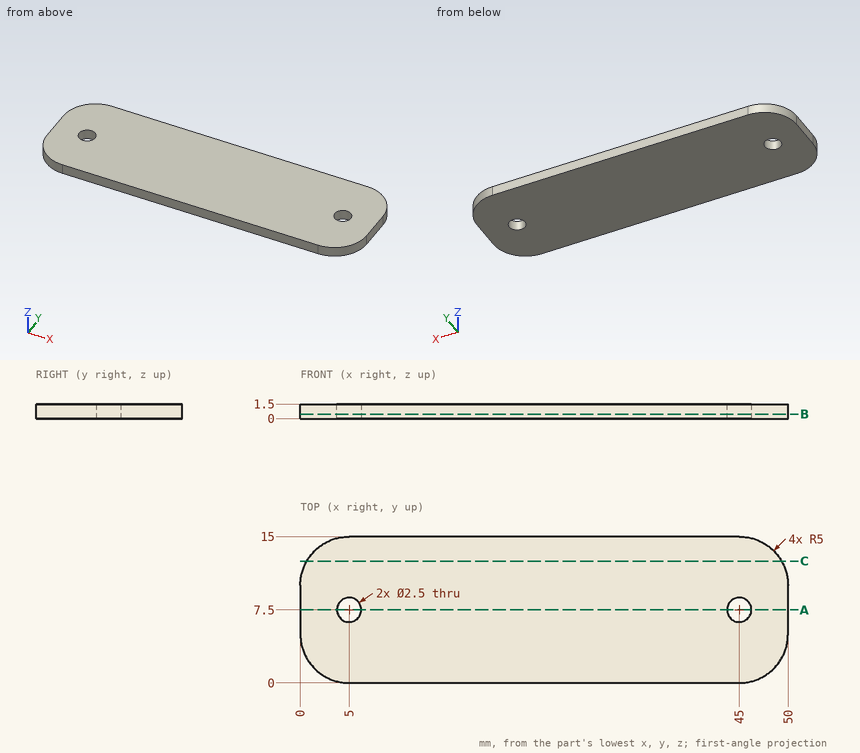
Check sheet for the drawn part. Datum: minimum x, y, z corner. Units: mm. Coordinates: 2 decimals unless noted, no trailing zeros. Loops run counter-clockwise (first coordinate to the right, second up) from the corner with the lowest first, then second, coordinate; pieces in that order, holes last. Notation, with made-up numbers: (35.5, -4) -> (69.5, -4) arc R26 cw to (69.5, 15) -> close; hole circle Ø8 at (73, 15). An arc over 180 degrees is marked (long way). Answer in a Markdown table with one row per item.
1) Section check B-B (z = 0.45). Record the cut outline in (x, y).
The answers:
| item | result |
|---|---|
| outline | (0, 5) arc R5 ccw to (5, 0) -> (45, 0) arc R5 ccw to (50, 5) -> (50, 10) arc R5 ccw to (45, 15) -> (5, 15) arc R5 ccw to (0, 10) -> close; hole circle Ø2.5 at (5, 7.5); hole circle Ø2.5 at (45, 7.5) |
2) Section check A-A (y = 7.5). Record the cut outline in (x, z), and give its area (3 significant figures).
The answers:
| item | result |
|---|---|
| outline | (0, 0) -> (3.75, 0) -> (3.75, 1.5) -> (0, 1.5) -> close; (6.25, 0) -> (43.75, 0) -> (43.75, 1.5) -> (6.25, 1.5) -> close; (46.25, 0) -> (50, 0) -> (50, 1.5) -> (46.25, 1.5) -> close |
| area | 67.5 mm2 |
3) Depth check by flat-ended pin: P1, Ø4, axis at x = 45, y = 7.5, coming from the -Z side; P2, Ø2, axis at x = 5, y = 7.5, coming from the +Z side. Enter the tip coordinate at first touch or a pass-through.
The answers:
| item | result |
|---|---|
| P1 | stops at z = 0 |
| P2 | passes through |
4) Scan lines: line 1 along Y through (x, z) = (45, 0.6); line 2 along X through (y, z) = (8, 1); line 3 along X through (y, z) = (6.75, 0.6). Record each from-to range of solid material in increasing order. Write a range as from..to.
The answers:
| item | result |
|---|---|
| line 1 | y = 0..6.25, 8.75..15 |
| line 2 | x = 0..3.85, 6.15..43.85, 46.15..50 |
| line 3 | x = 0..4, 6..44, 46..50 |
5) Section check C-C (y = 12.5). Record the cut outline in (x, z).
The answers:
| item | result |
|---|---|
| outline | (0.67, 0) -> (49.33, 0) -> (49.33, 1.5) -> (0.67, 1.5) -> close |
